Geometry: final body of the model. Coordinates: model frame, mm. A direction names the side the tool comes from. Round coordinates to 2 decimals unless told otherwise and drop trailing zeros. Order: outer loops, then holes, each group sorted by start corner. A loop starts at its lowest first (then second) coordinate and runs counter-clockwise, first axis right, second up. Notation, with made-up numbers: M 80,80.25 L 106,80.25 A29 cw 106,106.25 Z; hole C 36.25,28.25 d3. An arc over 180 degrees is marked long. Return JSON: item names as keys, results as strings. Group by question number.
Q1. Access query for faces 5 (the face through (22, 5, 29)), 6 (the face through (0, 19, 25)), 7 (the face through (22, -5, 29)), 8 (the face through (0, 0, 2)). Directions: +Z, -Z, +X, -X, +Y, -Y. A direction counts if a zero-diameter tool reaches every point of the face in a straight line with its end or side. Return the directions, or none.
Q2. Contact query for flat-ended pins moving along their axis: pin 1 (1.7 mm diameter, centred on y = 18, z = 27, fed in from -X); pin 2 (6 mm diameter, centred on y = -5.5, z = 11.5, fed in from +X); pin 3 (1.7 mm diameter, centred on y = 17.5, z = 27, fed in from +X). Output: stop coordinate, or through.
Q3. Cut plane B-B on z = 28.25. Output: boundary loops of the cut face in (x, y).
Q4. Ray query, probe 1 along Z at (x, y) = (22.5, 4); probe 2 along Y at (x, z) = (8.5, 8.75); probe 3 along Z at (x, y) = (-10, -7.5). Return the intervals inside material, ascending.
Q5. Cut plane D-D on z = 23.25. Output: boundary loops of the cut face in (x, y), and give its area (3 significant figures).
Q6. Cut plane A-A on y = 0. Output: boundary loops of the cut face in (x, z).
Q7. Cut plane C-C on x = 0. Output: boundary loops of the cut face in (y, z), and give its area (3 significant figures).
Q8. Mould query, pull axis X, two halves, no side actions, for faces 1 (the face through (7.5, 17, 28)), 2 (the face through (-26.64, 4.1, 28.48)), 3 (the face through (-3.902, -17.572, 16.196)), 4 (the face through (-22, -5, 29)). Classes: released by +X, released by -X, zero draft, split by the parting line, or undercut.
Autodesk Inventor part; units mm, degrees
ref_plane "YZ Plane" through (0, 0, 0) normal (1, 0, 0) x (0, 1, 0)
ref_plane "XZ Plane" through (0, 0, 0) normal (0, 1, 0) x (-1, 0, 0)
ref_plane "XY Plane" through (0, 0, 0) normal (0, 0, 1) x (1, 0, 0)
sketch "草圖1" plane through (0, 0, 0) normal (0, 0, 1) x (1, 0, 0)
  circle A0 centre (0, 0) radius 20
  dimension "d0" = 40
extrude "擠出1" add sketch "草圖1" along normal blind 30
sketch "草圖2" plane through (0, 0, 30) normal (0, 0, 1) x (1, 0, 0)
  circle A0 centre (0, 0) radius 18
  circle A1 centre (0, 0) radius 20
  dimension "d3" = 2
extrude "擠出2" cut sketch "草圖2" against normal blind 28 contours A0
sketch "草圖3" plane through (0, 0, 30) normal (0, 0, 1) x (1, 0, 0)
  line L0 (-7.5, 20) -> (7.5, 20)
  line L1 (7.5, 20) -> (7.5, 10)
  line L2 (7.5, 10) -> (-7.5, 10)
  line L3 (-7.5, 10) -> (-7.5, 20)
  circle A0 centre (0, 0) radius 20
  point P0 (0, 20)
  dimension "d6" = 15
  dimension "d7" = 10
extrude "擠出3" cut sketch "草圖3" against normal blind 5 contours L0 A0 L3 | L0 L1 A0 | A0 L1 L2 L3 picked at (0, 13.3333)
sketch "草圖4" plane through (0, 0, 30) normal (0, 0, 1) x (1, 0, 0)
  line L0 (-27.5, -5) -> (27.5, -5)
  line L1 (27.5, -5) -> (27.5, 5)
  line L2 (27.5, 5) -> (-27.5, 5)
  line L3 (-27.5, 5) -> (-27.5, -5)
  point P0 (0, 0)
  point P1 (0, -5)
  point P2 (-27.5, 0)
  dimension "d10" = 10
  dimension "d11" = 55
extrude "擠出4" add sketch "草圖4" against normal blind 3
sketch "草圖5" plane through (0, 0, 30) normal (0, 0, 1) x (1, 0, 0)
  circle A0 centre (0, 0) radius 18
  arc A1 (-17.2916, -5) -> (17.2916, -5) centre (0, 0) ccw
  dimension "d14" = 0
extrude "擠出5" cut sketch "草圖5" against normal up to surface (28 mm away)
sketch "草圖6" plane through (0, 0, 27) normal (0, 0, -1) x (-1, 0, 0)
  circle A0 centre (-24.5, 0) radius 1.6
  line L0 (-27.5, 5) -> (-27.5, -5)
  point P0 (0, 0)
  dimension "d17" = 3.2
  dimension "d18" = 3
extrude "擠出6" cut sketch "草圖6" against normal up to surface (3 mm away)
mirror "鏡射1" about plane through (0, 0, 0) normal (1, 0, 0) of "擠出6"
fillet "圓角1" radius 3 4 edges at (27.5, 5, 28.5) (27.5, -5, 28.5) (-27.5, 5, 28.5) (-27.5, -5, 28.5)
properties part number "音箱"
Result sheet:
{
 "1": {"face 5": "+Z, -Z, +X, +Y", "face 6": "+Z, +Y", "face 7": "+Z, -Z, +X, -Y", "face 8": "+Z"},
 "2": {"pin 1": "stops at x = -10.29", "pin 2": "stops at x = 19.84", "pin 3": "stops at x = 11.08"},
 "3": {"outline": "M -27.5,-2 A3 ccw -24.5,-5 L -19.36,-5 A20 ccw 19.36,-5 L 24.5,-5 A3 ccw 27.5,-2 L 27.5,2 A3 ccw 24.5,5 L 19.36,5 A20 ccw 7.5,18.54 L 7.5,16.36 A18 cw long -7.5,16.36 L -7.5,18.54 A20 ccw -19.36,5 L -24.5,5 A3 ccw -27.5,2 Z; hole C -24.5,0 d3.2; hole C 24.5,0 d3.2"},
 "4": {"probe 1": "z = 27 to 30", "probe 2": "y = -18.1 to -15.87, 15.87 to 18.1", "probe 3": "z = 0 to 2"},
 "5": {"outline": "C 0,0 d40; hole C 0,0 d36", "area": "239 mm²"},
 "6": {"outline": "M -27.5,27 L -26.1,27 L -26.1,30 L -27.5,30 Z; M -22.9,27 L -20,27 L -20,0 L 20,0 L 20,27 L 22.9,27 L 22.9,30 L 18,30 L 18,2 L -18,2 L -18,30 L -22.9,30 Z; M 26.1,27 L 27.5,27 L 27.5,30 L 26.1,30 Z"},
 "7": {"outline": "M -20,0 L 20,0 L 20,25 L 18,25 L 18,2 L -18,2 L -18,30 L -20,30 Z", "area": "182 mm²"},
 "8": {"face 1": "undercut", "face 2": "released by -X", "face 3": "undercut", "face 4": "zero draft"}
}
